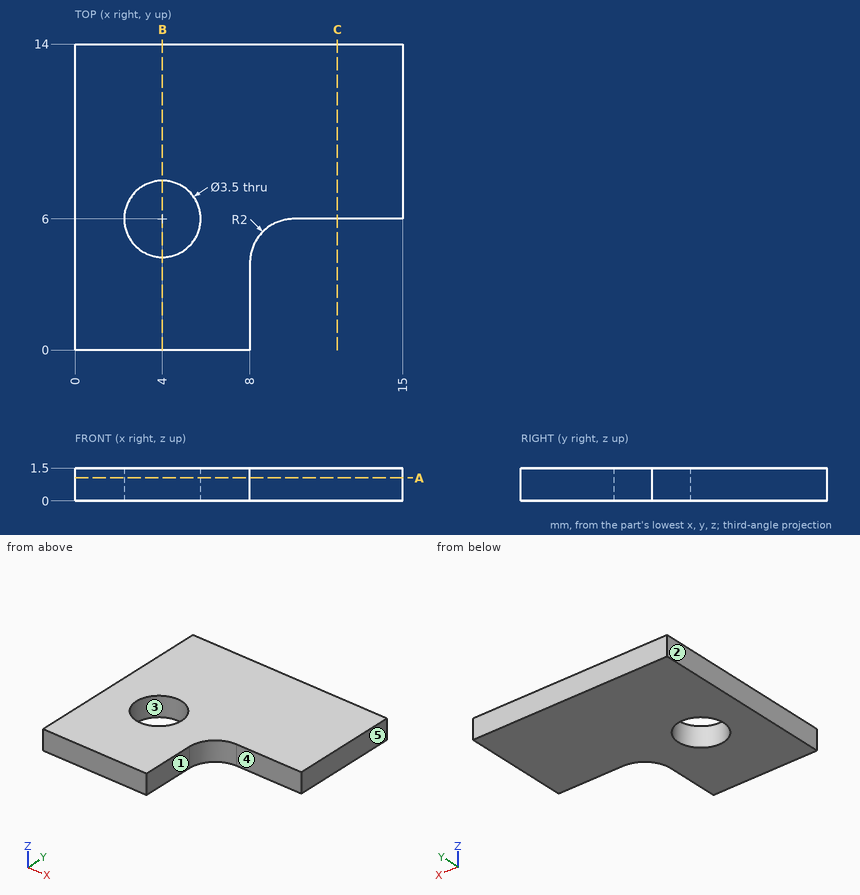
Input: dimensioned drawing with shaded views. Units: mm. Origin: part minimum x, y, z. A direction names the side the tool comes from. Round coordinates to 2 decimals unless told otherwise and drop trailing zeros. Loops run counter-clockwise (first coordinate to the right, second up) from the corner with the lowest first, then second, coordinate; pieces in that order, holes last. Notation, with made-up numbers: M 84.5,-24 L 113.5,-24 A26 ccw 113.5,13 Z; hole C 39,89.5 d1. An arc over 180 degrees is marked long. Return JSON: item names as keys, results as strings. Group by question number.
1. Mould query, pull axis Y, two halves, no side actions, for the marked faces 3, 4 and 5. Classes: released by +Y, released by -Y, zero draft, split by the parting line, or undercut.
2. Pin query (flat end, axial travel): pin 1 (1 mm diameter, centred on x = 12, y = 4, fed in from -Z). Return the tip coordinate at first contact, or that it passes through.
3. Section query C-C on x = 12. Output: boundary loops of the cut face in (y, z).
4. Material intervals for line 1 along Y through (x, z) = (4, 1); line 2 along X through (y, z) = (2, 1); line 3 along X through (y, z) = (5.5, 0.6), sorted ascending. Write a range as from..to.
5. Reachability of the marked faces 1 and 2 from +Z, -Z, +X, -X, +Y, -Y: full face, straight path, thin tool, end or side. Return the list, or none.
6. Section query B-B on x = 4. Output: boundary loops of the cut face in (y, z), and give its area (4 significant figures).
7. Section query A-A on z = 1.05. Output: boundary loops of the cut face in (x, y), and give its area (3 significant figures).
Checks:
{
 "1": {"face 3": "undercut", "face 4": "released by -Y", "face 5": "zero draft"},
 "2": {"pin 1": "passes through"},
 "3": {"outline": "M 6,0 L 14,0 L 14,1.5 L 6,1.5 Z"},
 "4": {"line 1": "y = 0..4.25, 7.75..14", "line 2": "x = 0..8", "line 3": "x = 0..2.32, 5.68..8.68"},
 "5": {"face 1": "+Z, -Z, +X, -Y", "face 2": "+Z, -Z, -X, +Y, -Y"},
 "6": {"outline": "M 0,0 L 4.25,0 L 4.25,1.5 L 0,1.5 Z; M 7.75,0 L 14,0 L 14,1.5 L 7.75,1.5 Z", "area": "15.75 mm²"},
 "7": {"outline": "M 0,0 L 8,0 L 8,4 A2 cw 10,6 L 15,6 L 15,14 L 0,14 Z; hole C 4,6 d3.5", "area": "159 mm²"}
}
